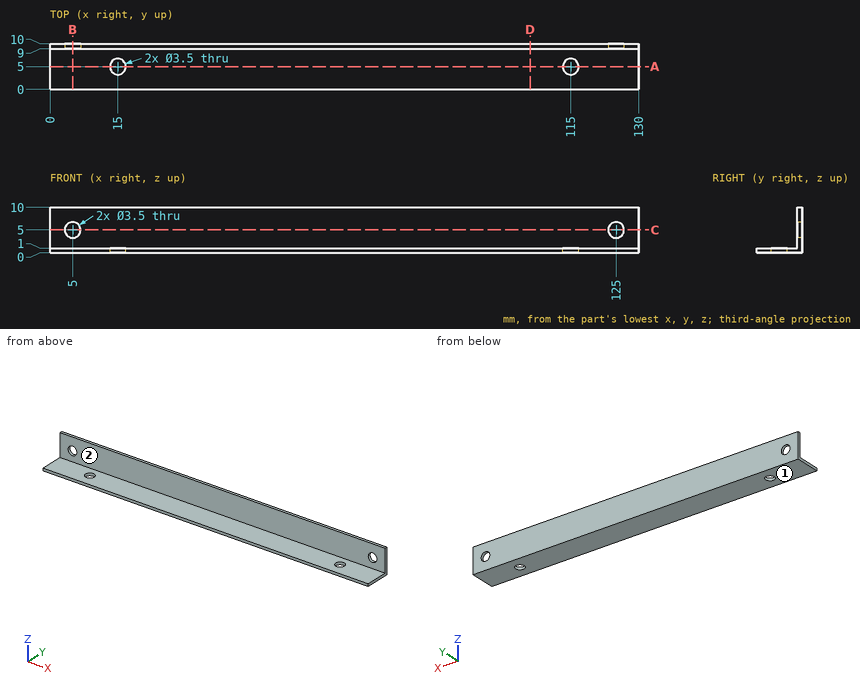
Answer from the drawing. Dimensions are ordinates in mm from the lowest x, y and z of the part. A direction names the side the tool comes from. Round coordinates to 2 decimals unless told otherwise and drop trailing zeros. Loops run counter-clockwise (first coordinate to the right, second up) from the corner with the lowest first, then second, coordinate; pieces in that order, holes last.
Q1. Which of the six approach directions +Z, -Z, +X, -X, +Y, -Y give full straight-line access (tool end or side, diameter ignored) to the marked faces 1 and 2?
Q2. Section C-C on z = 5 is taken. Write down the section's boundary in (x, y).
Q3. Section A-A on y = 5 is taken. Write down the section's boundary in (x, z), and give its area (3 significant figures).
Q4. Consider probe 1 along X at (y, z) = (5, 0.6); probe 2 along Z at (x, y) = (125, 9.55). Determine where each line is inside the solid, lowest interval first.
Q5. Section B-B on x = 5 is taken. Write down the section's boundary in (y, z).
Q6. Each of these flat-tipped pins is pushed along its axis until it touches: pin 1 (2.5 mm diameter, centred on x = 71.5, z = 6.5, fed in from -Y); pin 2 (4.5 mm diameter, centred on x = 36, y = 6.5, fed in from +Z). Where does it stop, or does it pass through?
Q7. Section D-D on x = 106 is taken. Write down the section's boundary in (y, z), and give its area (3 significant figures).
Output:
1. face 1: -Z, +X, -X, +Y, -Y
1. face 2: +Z, +X, -X, -Y
2. outline: (0, 9) - (3.25, 9) - (3.25, 10) - (0, 10) - close; (6.75, 9) - (123.25, 9) - (123.25, 10) - (6.75, 10) - close; (126.75, 9) - (130, 9) - (130, 10) - (126.75, 10) - close
3. outline: (0, 0) - (13.25, 0) - (13.25, 1) - (0, 1) - close; (16.75, 0) - (113.25, 0) - (113.25, 1) - (16.75, 1) - close; (116.75, 0) - (130, 0) - (130, 1) - (116.75, 1) - close
3. area: 123 mm2
4. probe 1: x = 0 to 13.25, 16.75 to 113.25, 116.75 to 130
4. probe 2: z = 0 to 3.25, 6.75 to 10
5. outline: (0, 0) - (10, 0) - (10, 3.25) - (9, 3.25) - (9, 1) - (0, 1) - close; (9, 6.75) - (10, 6.75) - (10, 10) - (9, 10) - close
6. pin 1: stops at y = 9
6. pin 2: stops at z = 1
7. outline: (0, 0) - (10, 0) - (10, 10) - (9, 10) - (9, 1) - (0, 1) - close
7. area: 19.0 mm2
